Can you work these out from the model? Positions are in its coordinate system, mm. Round coordinates to 2 decimals unless told otherwise and drop trailing zeros. Write each loop counter-clockwise with the first axis right and the second up, starting at its lowest first coordinate (ties: lowest second). Pieces come first, ordered by that corner, then holes. Notation, with made-up numbers: (77, -22.5) -> (120, -22.5) arc R32 ccw to (120, 8.5) -> close; hole circle Ø3 at (58.25, 44). An arc over 180 degrees is marked (long way). Use CSV: the item, a comma, the result in double quotes.
Autodesk Inventor part; units mm, degrees
ref_plane "YZ Plane" through (0, 0, 0) normal (1, 0, 0) x (0, 1, 0)
ref_plane "XZ Plane" through (0, 0, 0) normal (0, 1, 0) x (-1, 0, 0)
ref_plane "XY Plane" through (0, 0, 0) normal (0, 0, 1) x (1, 0, 0)
sketch "Sketch8" plane through (0, 0, 0) normal (0, 0, 1) x (1, 0, 0)
  line L0 (-3, 0) -> (-3, 3)
  line L1 (0, 0) -> (444, 0)
  line L2 (444, 0) -> (444, 3)
  line L3 (0, 3) -> (444, 3)
  line L4 (0, 0) -> (0, 3)
  line L5 (0, 3) -> (-3, 3)
  line L6 (0, 0) -> (-3, 0)
  line L7 (447, 3) -> (444, 3)
  line L8 (447, 0) -> (447, 3)
  line L9 (447, 0) -> (444, 0)
  line L10 (0, 4.5) -> (442, 4.5)
  line L11 (0, -1.5) -> (442, -1.5)
  line L12 (442, 4.5) -> (442, -1.5)
  line L13 (2, 4.5) -> (2, -1.5)
  line L14 (2, 4.5) -> (442, 4.5)
  line L15 (442, 4.5) -> (442, 11.5)
  line L16 (442, 11.5) -> (2, 11.5)
  line L17 (2, 11.5) -> (2, 4.5)
  line L18 (2, -1.5) -> (442, -1.5)
  line L19 (442, -1.5) -> (442, -8.5)
  line L20 (442, -8.5) -> (2, -8.5)
  line L21 (2, -8.5) -> (2, -1.5)
  point P0 (-3, 1.5)
extrude "Extrusion7" add sketch "Sketch8" along normal blind 6 contours L11 L19 L20 L21 | L17 L16 L15 L10
sketch "Sketch9" plane through (0, 0, 6) normal (0, 0, 1) x (1, 0, 0)
  line L0 (2, 11.5) -> (2, 4.5)
  line L1 (2, 4.5) -> (442, 4.5)
  line L2 (442, 4.5) -> (442, 11.5)
  line L3 (442, 11.5) -> (2, 11.5)
  line L4 (442, -8.5) -> (442, -1.5)
  line L5 (442, -1.5) -> (2, -1.5)
  line L6 (2, -1.5) -> (2, -8.5)
  line L7 (2, -8.5) -> (442, -8.5)
  line L8 (2, 4.5) -> (2, -1.5)
  line L9 (442, -1.5) -> (442, 4.5)
  point P0 (0, 0)
extrude "Extrusion8" add sketch "Sketch9" along normal blind 1
sketch "Sketch10" plane through (0, 0, 7) normal (0, 0, 1) x (1, 0, 0)
  line L0 (2, 4.5) -> (442, 4.5)
  line L1 (442, -1.5) -> (2, -1.5)
  line L2 (442, -2.5) -> (2, -2.5)
  line L3 (2, 5.5) -> (442, 5.5)
  line L4 (2, 5.5) -> (2, -2.5)
  line L5 (2, 11.5) -> (2, -8.5)
  line L6 (442, 5.5) -> (442, -2.5)
  point P0 (0, 0)
  dimension "d33" = 1
  dimension "d34" = 1
extrude "Extrusion9" add sketch "Sketch10" along normal blind 6
sketch "Sketch11" plane through (0, 0, 13) normal (0, 0, 1) x (1, 0, 0)
  line L0 (447, 0) -> (444, 0)
  line L1 (2, 5.5) -> (442, 5.5)
  line L2 (442, 5.5) -> (442, 11.5)
  line L3 (442, 11.5) -> (2, 11.5)
  line L4 (2, 11.5) -> (2, 5.5)
  line L5 (442, -2.5) -> (2, -2.5)
  line L6 (2, -2.5) -> (2, -8.5)
  line L7 (2, -8.5) -> (442, -8.5)
  line L8 (442, -8.5) -> (442, -2.5)
  line L9 (442, 5.5) -> (2, 5.5)
  line L10 (2, 5.5) -> (2, -2.5)
  line L11 (2, -2.5) -> (442, -2.5)
  line L12 (442, -2.5) -> (442, 5.5)
  point P0 (0, 0)
  point P1 (2, -2.5)
extrude "Extrusion10" add sketch "Sketch11" along normal blind 1
sketch "Sketch12" plane through (0, 0, 14) normal (0, 0, 1) x (1, 0, 0)
  line L0 (442, 5.5) -> (2, 5.5)
  line L1 (2, 11.5) -> (2, 4.5)
  line L2 (442, 11.5) -> (2, 11.5)
  line L3 (442, 4.5) -> (442, 11.5)
  line L4 (2, 4.5) -> (442, 4.5)
  line L5 (442, -8.5) -> (442, -1.5)
  line L6 (2, -8.5) -> (442, -8.5)
  line L7 (2, -1.5) -> (2, -8.5)
  line L8 (442, -1.5) -> (2, -1.5)
  point P0 (0, 0)
extrude "Extrusion11" add sketch "Sketch12" along normal blind 6
properties part number "xbar"
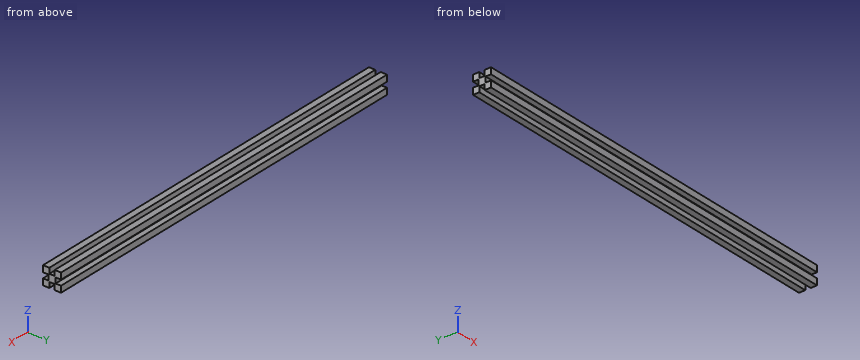
Q1. Suppose I cut it at B-B (z = 17). Write out the boundary of the cut face in (x, y).
Resolved:
outline,"(2, -8.5) -> (442, -8.5) -> (442, -1.5) -> (2, -1.5) -> close; (2, 4.5) -> (442, 4.5) -> (442, 11.5) -> (2, 11.5) -> close"
Q2. Will these pins go through, and if not, where does the flat tip stop? P1, Ø5, axis at x = 196, y = 2.5, coming from the -Z side; P2, Ø1.8, axis at x = 290.5, z = 11, coming from the +Y side; P3, Ø1.5, axis at y = 3, z = 4.5, coming from the +X side.
Resolved:
P1,"stops at z = 0"
P2,"stops at y = 5.5"
P3,"passes through"
Q3. Suppose I cut it at C-C (x = 271). Write out the boundary of the cut face in (y, z), and give its area (3 significant figures).
Resolved:
outline,"(-8.5, 0) -> (-1.5, 0) -> (-1.5, 6) -> (4.5, 6) -> (4.5, 0) -> (11.5, 0) -> (11.5, 7) -> (5.5, 7) -> (5.5, 13) -> (11.5, 13) -> (11.5, 20) -> (4.5, 20) -> (4.5, 14) -> (-1.5, 14) -> (-1.5, 20) -> (-8.5, 20) -> (-8.5, 13) -> (-2.5, 13) -> (-2.5, 7) -> (-8.5, 7) -> close"
area,"256 mm^2"
Q4. Suppose I cut it at A-A (y = 8.5). Write out the boundary of the cut face in (x, z), and give its area (3 significant figures).
Resolved:
outline,"(2, 0) -> (442, 0) -> (442, 7) -> (2, 7) -> close; (2, 13) -> (442, 13) -> (442, 20) -> (2, 20) -> close"
area,"6,160 mm^2"
Q5. Please list where these lines run through material, in increasing order: probe 1 along Y at (x, z) = (303, 16.5); probe 2 along Z at (x, y) = (115, 6); probe 3 along Z at (x, y) = (292, 1).
Resolved:
probe 1,"y = -8.5 to -1.5, 4.5 to 11.5"
probe 2,"z = 0 to 7, 13 to 20"
probe 3,"z = 6 to 14"
